Here's how the part is built. I have some questions about the finished solid (model axes, mm). Face numbers are marked on the shaded views. A direction names the side the tool comes from. Give positions to 0.01 mm unless a question says otherwise; leave off trailing zeros. Order: outer loops, then holes, each group sorted by start corner. A loop starts at its lowest first (then second) coordinate and runs counter-clockwise, first axis right, second up. Notation, with made-up numbers: (53, 53) -> (80, 53) arc R21 cw to (80, 61) -> close; hole circle Ø10 at (-9.75, 80). An arc over 180 degrees is marked (long way). Write each question's results on one line, items separated by ' | '. Start each with the question number.
Q1. For the marked faces 1, 2 and 3, which set-ups out of +Z, -Z, +X, -X, +Y, -Y let a thin tool reach every point of the face, with its end or its side?
Q2. I need wall thicknesses on line 1 along Y through (x, z) = (-23.5, 1.75); line 2 along Y through (x, z) = (-16, 23.75); line 3 along Z through (x, y) = (-20.5, -22). Which ranges of each line are inside material? Lowest first, please. Write a range as [from, to].
Q3. I'm going to push flat-ended pins straight in: pin 1 (2 mm diameter, centred on y = -31, z = 9, fed in from -X); pin 2 (1.5 mm diameter, centred on x = -10.5, y = -12, fed in from +Z); pin 3 (6 mm diameter, centred on x = -9.5, z = 20.5, fed in from -Y). Where does each tip first touch, or does it pass through?
Q4. Imagine slicing it at C-C, the plane y = -3. Please give me the cut outline in (x, z), then the cut area to 3 significant figures.
Q5. Imagine slicing it at A-A, the plane z = 26. Please give me the cut outline in (x, y), then the cut area to 3 significant figures.
Q6. Imagine slicing it at B-B, the plane x = -25.5. Please give me the cut outline in (y, z), then the cut area to 3 significant figures.
Q7. Imagine slicing it at D-D, the plane z = 15.5. Please give me the cut outline in (x, y), then the cut area to 3 significant figures.
Q8. Thinking about a two-plate mould opening in X: for the marked faces 4, 5 and 6, which applies, pulls with the +X half, pulls with the -X half, needs draft (parallel to the pull), parting line crosses it, or undercut?
```python
from build123d import *

# Parameters (mm, degrees)
F1_DEPTH  = 30
F2_W      = 11
F2_H      = 15
F3_DEPTH  = 11
F4_W      = 15
F4_H      = 8
F5_DEPTH  = 11
F6_ANGLE  = -90
F8_DEPTH  = 11
F10_DEPTH = 11


with BuildPart() as f1:
    # F0 (on Front) → F1 (new body)
    with BuildSketch(Plane.XZ):
        Polygon((0, 30), (0, 0), (40, 0), (40, 11), (11, 11), (11, 30), align=None)
    extrude(amount=F1_DEPTH)

    # F2 (on face) → F3 (cut, through all)
    with BuildSketch(Plane.XY.offset(11)):
        with Locations((34.5, -22.5)):
            Rectangle(F2_W, F2_H)
    extrude(amount=-F3_DEPTH, mode=Mode.SUBTRACT)

    # F4 (on face) → F5 (cut, through all)
    with BuildSketch(Plane.YZ.offset(11)):
        with Locations((-22.5, 26)):
            Rectangle(F4_W, F4_H)
    extrude(amount=-F5_DEPTH, mode=Mode.SUBTRACT)


with BuildPart() as f1_1:
    # F6: moved
    add(f1.part.rotate(Axis((0, 0, 15), (0, 0, 1)), F6_ANGLE))

    # F7 (on face) → F8 (join, through all)
    with BuildSketch(Plane.XZ.offset(11)):
        Polygon((-15, 22), (-15, 30), (-30, 22), align=None)
    extrude(amount=-F8_DEPTH)

    # F9 (on face) → F10 (cut, through all)
    with BuildSketch(Plane.XZ.offset(11)):
        Polygon((0, 30), (-15, 30), (-15, 22), align=None)
    extrude(amount=-F10_DEPTH, mode=Mode.SUBTRACT)


solid = f1_1.part
```
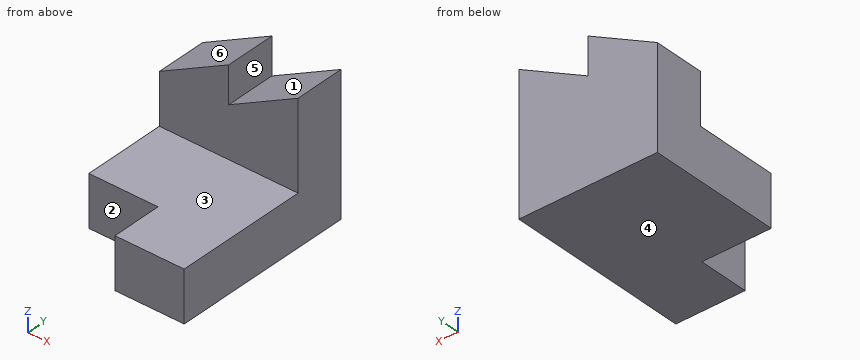
Geometry check:
1) face 1: +Z, +Y, -Y | face 2: +Z, -Z, -X, -Y | face 3: +Z, +X, -X, -Y
2) line 1: [-29, 0] | line 2: [-11, 0] | line 3: [0, 11]
3) pin 1: x = -15 | pin 2: z = 11 | pin 3: y = -11
4) outline: (-30, 0) -> (0, 0) -> (0, 30) -> (-15, 22) -> (-15, 30) -> (-30, 22) -> close | area: 780 mm²
5) outline: (-22.5, -11) -> (-15, -11) -> (-15, 0) -> (-22.5, 0) -> close; (-7.5, -11) -> (0, -11) -> (0, 0) -> (-7.5, 0) -> close | area: 165 mm²
6) outline: (-29, 0) -> (0, 0) -> (0, 24.4) -> (-11, 24.4) -> (-11, 11) -> (-29, 11) -> close | area: 466 mm²
7) outline: (-30, -11) -> (0, -11) -> (0, 0) -> (-30, 0) -> close | area: 330 mm²
8) face 4: needs draft | face 5: undercut | face 6: pulls with the -X half
